Geometry check sheet. Reference: the model listing, model coordinates, mm. A direction names the side the tool comes from. Coordinates: 2 decimals unless noted, no trailing zeros. Order: outer loops, then holes, each group sorted by start corner. A loop starts at its lowest first (then second) coordinate and runs counter-clockwise, first axis right, second up. Notation, with made-up numbers: (55, 48.5) - (108, 48.5) arc R18 ccw to (108, 54.5) - close; hole circle Ø1 at (88.25, 35). An arc over 180 degrees is marked (long way). Put each result on its own line as item: value.
from build123d import *

# Parameters (mm, degrees)
F0_W      = 15.6
F0_H      = 11
F1_DEPTH  = 23.2
F3_DEPTH  = 25
F4_R      = 2.5
F5_DEPTH  = 3.2
F6_R      = 2.2
F7_DEPTH  = 3
F8_R      = 2.2
F9_DEPTH  = 3
F10_R     = 2.5
F11_DEPTH = 3
F13_R     = 2.2
F14_DEPTH = 3
F12_R     = 2.5
F15_DEPTH = 3.2
F16_R     = 2.5
F18_DEPTH = 3.2
F17_R     = 2.2
F19_DEPTH = 3


# Not quite as in the source:
# - a feature names something its author has since deleted; it is built from what else it names


with BuildPart() as f1:
    # F0 (on Top) → F1 (new body)
    with BuildSketch(Plane.XY):
        with Locations((-7.8, 0)):
            Rectangle(F0_W, F0_H)
        with Locations((7.8, 0)):
            Rectangle(F0_W, F0_H)
    extrude(amount=F1_DEPTH)

    # F2 (on face) → F3 (cut)
    with BuildSketch(Plane.XZ.offset(5.5)):
        Polygon((0, 18.2), (-11, 18.2), (-11, 5.6), (-6, 5.6), (-6, 9.1), (0, 9.1), (6, 9.1), (6, 5.6), (11, 5.6), (11, 18.2), align=None)
    extrude(amount=-F3_DEPTH, mode=Mode.SUBTRACT)

    # F4 (on face) → F5 (cut)
    with BuildSketch(Plane(origin=(0, 0, 0), x_dir=(1, 0, 0), z_dir=(0, 0, -1))):
        with Locations((-7.8, 0)):
            Circle(F4_R)
    extrude(amount=-F5_DEPTH, mode=Mode.SUBTRACT)

    # F6 (on face) → F7 (join)
    with BuildSketch(Plane(origin=(0, 0, 0), x_dir=(1, 0, 0), z_dir=(0, 0, -1))):
        with Locations((7.8, 0)):
            Circle(F6_R)
    extrude(amount=F7_DEPTH)

    # F8 (on face) → F9 (join)
    with BuildSketch(Plane.XY.offset(23.2)):
        with Locations((-7.8, 0)):
            Circle(F8_R)
    extrude(amount=F9_DEPTH)

    # F10 (on face) → F11 (cut)
    with BuildSketch(Plane.XY.offset(23.2)):
        with Locations((7.8, 0)):
            Circle(F10_R)
    extrude(amount=-F11_DEPTH, mode=Mode.SUBTRACT)

    # F13 (on face) → F14 (join)
    with BuildSketch(Plane.YZ.offset(15.6)):
        with Locations((0, 16.5)):
            Circle(F13_R)
    extrude(amount=F14_DEPTH)

    # F12 (on face) → F15 (cut)
    with BuildSketch(Plane.YZ.offset(15.6)):
        with Locations((0, 7)):
            Circle(F12_R)
    extrude(amount=-F15_DEPTH, mode=Mode.SUBTRACT)

    # F16 (on face) → F18 (cut)
    with BuildSketch(Plane(origin=(-15.6, 0, 0), x_dir=(0, -1, 0), z_dir=(-1, 0, 0))):
        with Locations((0, 16.5)):
            Circle(F16_R)
    extrude(amount=-F18_DEPTH, mode=Mode.SUBTRACT)

    # F17 (on face) → F19 (join)
    with BuildSketch(Plane(origin=(-15.6, 0, 0), x_dir=(0, -1, 0), z_dir=(-1, 0, 0))):
        with Locations((0, 7)):
            Circle(F17_R)
    extrude(amount=F19_DEPTH)


solid = f1.part
Q1. Section check A-A on y = 3.25. Record the boundary of the cut face in (x, z), then the cut area to 3 significant figures.
Answer block:
outline: (-15.6, 0) - (15.6, 0) - (15.6, 23.2) - (-15.6, 23.2) - close; hole (-11, 5.6) - (-6, 5.6) - (-6, 9.1) - (6, 9.1) - (6, 5.6) - (11, 5.6) - (11, 18.2) - (-11, 18.2) - close
area: 489 mm^2
Q2. Depth check by flat-ended pin: pin 1 Ø3 at (y, z) = (3.5, 20.5) entering from -X; pin 2 Ø1.5 at (x, y) = (7.5, 0) entering from +Z; pin 3 Ø4.5 at (y, z) = (0, 7) entering from +X. Enter the tip coordinate at first touch or a pass-through.
Answer block:
pin 1: stops at x = -15.6
pin 2: stops at z = 20.2
pin 3: stops at x = 12.4
Q3. Access from +Z, -Z, +X, -X, +Y, -Y to the whole of each face (thin tool, end or side, straight path). Record for faces 1 (the flat face through (-12.4, 0, 17)), 2 (the flat face through (-9, 0, 5.6)), 3 (the cylindrical face through (14.02, -0.54, 4.56)), 4 (the flat face through (8, 0, 20.2)).
Answer block:
face 1: -X
face 2: +Y, -Y
face 3: +X
face 4: +Z
Q4. Thickness scan on L1, parallel to X at y = -1, z = 6; L2, parallel to Z at x = -10.5, y = -4.5; L3, parallel to X at y = 4, z = 14. Record the ranges inside material, lowest first. Write a range as [from, to].
Answer block:
L1: x = [-18.6, -11], [-6, 6], [11, 12.4]
L2: z = [0, 5.6], [18.2, 23.2]
L3: x = [-15.6, -11], [11, 15.6]
Q5. Draft check along Z on faces 5 (the flat face through (8, 0, 5.6)), 6 (the flat face through (15.6, 0, 11)), 7 (the cylindrical face through (17.079, -0.477, 14.352)). Enter one of: pulls with the +Z half, pulls with the -Z half, needs draft (parallel to the pull), parting line crosses it, or undercut.
Answer block:
face 5: undercut
face 6: needs draft
face 7: parting line crosses it
Q6. Section check D-D on z = 16.5. Record the boundary of the cut face in (x, y).
Answer block:
outline: (-15.6, -5.5) - (-11, -5.5) - (-11, 5.5) - (-15.6, 5.5) - (-15.6, 2.5) - (-12.4, 2.5) - (-12.4, -2.5) - (-15.6, -2.5) - close; (11, -5.5) - (15.6, -5.5) - (15.6, -2.2) - (18.6, -2.2) - (18.6, 2.2) - (15.6, 2.2) - (15.6, 5.5) - (11, 5.5) - close
Q7. Section check C-C on z = 2.25. Record the boundary of the cut face in (x, y), then the cut area to 3 significant figures.
Answer block:
outline: (-15.6, -5.5) - (15.6, -5.5) - (15.6, 5.5) - (-15.6, 5.5) - close; hole circle Ø5 at (-7.8, 0)
area: 324 mm^2
Q8. Section check B-B on x = 7.8. Record the boundary of the cut face in (y, z).
Answer block:
outline: (-5.5, 0) - (-2.2, 0) - (-2.2, -3) - (2.2, -3) - (2.2, 0) - (5.5, 0) - (5.5, 5.6) - (-5.5, 5.6) - close; (-5.5, 18.2) - (5.5, 18.2) - (5.5, 23.2) - (2.5, 23.2) - (2.5, 20.2) - (-2.5, 20.2) - (-2.5, 23.2) - (-5.5, 23.2) - close
